Read the model definition and answer for the solid it produces. Units are mm, in the model's axes. A direction names the side the tool comes from. Coordinates: 2 decimals unless noted, no trailing zeros. Write each loop counter-clockwise with the first axis right and the second up, starting at its lowest first coordinate (ties: lowest second). Pieces come first, ordered by that corner, then holes. Notation, with made-up numbers: (-33, 6) - (17, 6) arc R18 ccw to (17, 25) - close; hole circle Ø5 at (63.25, 29.25). An arc over 180 degrees is marked (long way). Return JSON: item names as keys, results as strings.
```python
from build123d import *

# Parameters (mm, degrees)
FILLET1_R = 160


with BuildPart() as part:
    # Sketch1 → Revolve1 (revolve)
    with BuildSketch(Plane(origin=(0, 0, 0), x_dir=(0, 0, -1), z_dir=(1, 0, 0)), mode=Mode.PRIVATE) as revolve1_sk:
        Polygon((140, 159.946981615), (145, 159.946981615), (145, 119.946981615), (125, 64.997433226), (125, -45.002566774), (106.801488287, -95.002566774), (101.801488287, -95.002566774), (120, -45.002566774), (120, -15.087139211), (121, -15.087139211), (121, 54.912860789), (120, 54.912860789), (120, 64.997433226), (140, 119.946981615), align=None)
    revolve(revolve1_sk.sketch.rotate(Axis((0, 159.946981615, 0), (0, -1, 0)), 180), axis=Axis((0, 159.946981615, 0), (0, -1, 0)))

    # Fillet1
    fillet1_edges = [part.edges().sort_by_distance(p)[0] for p in [
        (0, -45.002566774, -125),
        (0, 64.997433226, -125),
        (0, 119.946981615, -145),
    ]]
    fillet(fillet1_edges, radius=FILLET1_R)


solid = part.part
```
(1) A cutting plane is placed at A-A (y = 29). Determine the outline of the cut face in (x, z), and give its area (3 significant figures).
Answer:
{"outline": "circle Ø250 at (0, 0); hole circle Ø242 at (0, 0)", "area": "3,090 mm²"}
(2) Flat-ended cylindrical pins translate along their axes: P1, Ø1.5, axis at y = 6.5, z = 107, coming from the -X side; P2, Ø1.5, axis at y = -5, z = -3, coming from the +X side; P3, Ø3, axis at x = -110.5, y = 129, coming from the -Z side. Find the tip coordinate at first contact, or state that the pin passes through.
Answer:
{"P1": "x = -65.85", "P2": "x = 124.98", "P3": "z = -93.89"}
(3) Determine the mould class of faces 1 (the face through (-102.064, -91.875, -13.401)), 2 (the face through (-119, 159.947, 76)), 3 (the face through (118.368, 68.435, -26.285)), 4 (the face through (95.12, -93.862, 49.474)) for opening direction Z: +Z half, -Z half, draft (parallel to the pull), parting line (faces both ways), or undercut.
Answer:
{"face 1": "undercut", "face 2": "draft", "face 3": "undercut", "face 4": "parting line"}
(4) Straight lines are drawn through the part: line 1 (X direction, y = 151, z = 0); line 2 (X direction, y = 27, z = 0); line 3 (Z direction, x = 109.5, y = 33.5). For each, find the intervals that lie inside material, in ascending order. Write a range as from..to.
Answer:
{"line 1": "-145..-140, 140..145", "line 2": "-125..-121, 121..125", "line 3": "-60.29..-51.49, 51.49..60.29"}
(5) A cutting plane is placed at B-B (y = -78.5). Determine the outline of the cut face in (x, z).
Answer:
{"outline": "circle Ø225.62 at (0, 0); hole circle Ø215.62 at (0, 0)"}
(6) Which of the six approach directions +Z, -Z, +X, -X, +Y, -Y give full straight-line access (tool end or side, diameter ignored) to faces 5 (the face through (128.64, 153.97, 66.91)), 6 (the face through (94.4, -95.003, 39.1)), 7 (the face through (-27.5, 54.913, -117.1)), 8 (the face through (-37.547, 9.622, 119.228)), 9 (the face through (-101.184, -29.835, 64.511))?
Answer:
{"face 5": "+Y, -Y", "face 6": "+Z, -Z, +X, -X, -Y", "face 7": "none", "face 8": "-Y", "face 9": "+Y"}
